Could you check a few things on this drawing? It's one solid part, dimensions in mm from its lowest x, y, z. Give positions to 0.01 mm unless a question says otherwise; leave off trailing zeros. Loops run counter-clockwise (first coordinate to the right, second up) from the corner with the lowest first, then second, coordinate; pieces in that order, holes last. Notation, with made-up numbers: M -19.75,27.25 L 25.25,27.25 A33 ccw 25.25,63.25 Z; hole C 87,59.25 d3. An arc over 180 degrees is marked long. Answer as a JSON object with one key per item and string values.
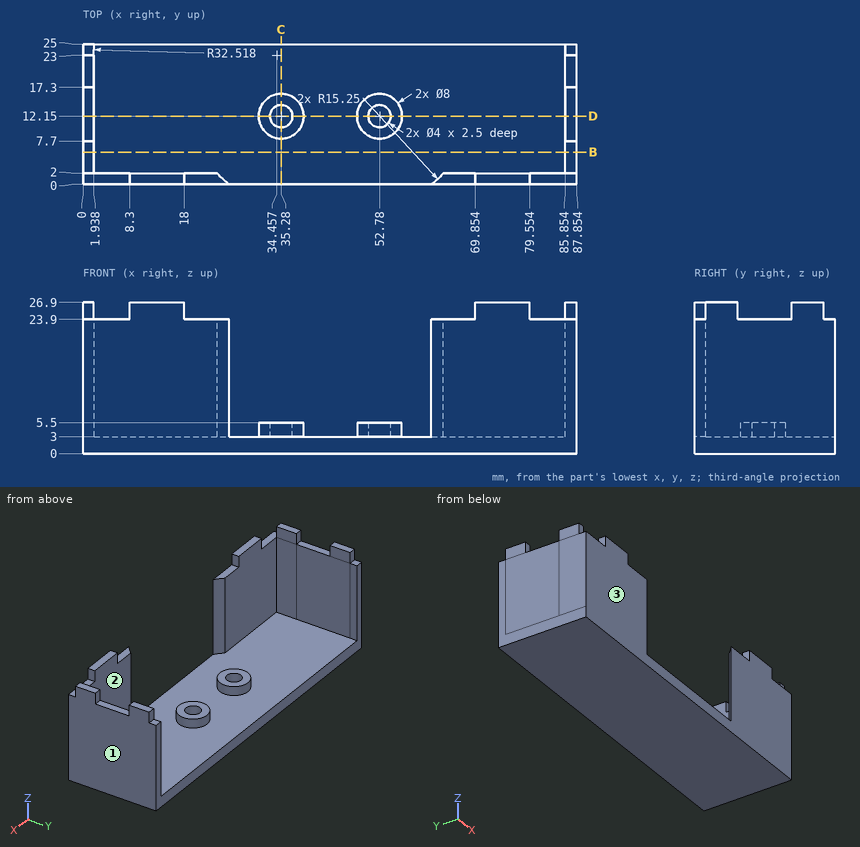
1) Suppose I cut it at C-C, the plane x = 35.28. Write out the boundary of the cut face in (y, z).
Answer list:
{"outline": "M 0,0 L 25,0 L 25,3 L 16.15,3 L 16.15,5.5 L 14.15,5.5 L 14.15,3 L 10.15,3 L 10.15,5.5 L 8.15,5.5 L 8.15,3 L 0,3 Z"}
2) Please list where these lines run through material, in increasing order: line 1 along X through (y, z) = (5.5, 17) (1 decimal); line 2 along Y through (x, z) = (52.78, 4.55); line 3 along Z through (x, y) = (80, 8). Write a range as from..to.
Answer list:
{"line 1": "0..1.9, 85.9..87.9", "line 2": "8.15..10.15, 14.15..16.15", "line 3": "0..3"}
3) If we mould it in two halves opening along X, with no side actions, what happens to the marked faces 1, 2 and 3? For each: +X half, -X half, draft (parallel to the pull), parting line (faces both ways), or undercut.
Answer list:
{"face 1": "+X half", "face 2": "undercut", "face 3": "draft"}
4) Suppose I cut it at B-B, the plane y = 5.75. Write out the boundary of the cut face in (x, z) (1 decimal).
Answer list:
{"outline": "M 0,0 L 87.9,0 L 87.9,26.9 L 85.9,26.9 L 85.9,3 L 1.9,3 L 1.9,26.9 L 0,26.9 Z"}
5) Will these pins go through, and if not, where does the flat tip stop? pin 1 Ø4.5 at (x, y) = (53.5, 12) entering from +Z; pin 2 Ø2 at (x, y) = (87, 11.5) entering from +Z; pin 3 Ø0.6 at (x, z) = (87, 25.5) entering from +Y.
Answer list:
{"pin 1": "z = 5.5", "pin 2": "z = 23.9", "pin 3": "y = 23"}
6) Suppose I cut it at D-D, the plane y = 12.15. Write out the boundary of the cut face in (x, z) (1 decimal).
Answer list:
{"outline": "M 0,0 L 87.9,0 L 87.9,23.9 L 85.9,23.9 L 85.9,3 L 56.8,3 L 56.8,5.5 L 54.8,5.5 L 54.8,3 L 50.8,3 L 50.8,5.5 L 48.8,5.5 L 48.8,3 L 39.3,3 L 39.3,5.5 L 37.3,5.5 L 37.3,3 L 33.3,3 L 33.3,5.5 L 31.3,5.5 L 31.3,3 L 1.9,3 L 1.9,23.9 L 0,23.9 Z"}
